Read the model definition and answer for the solid it produces. Units are mm, in the model's axes. Face numbers are marked on the shaded views. A direction names the side the tool comes from. Coordinates: 2 decimals unless noted, no trailing zeros. Write each loop counter-clockwise with the first axis right and the second up, starting at its lowest first coordinate (ties: lowest second). Pieces come first, ordered by that corner, then holes. Notation, with made-up numbers: (42, 24) -> (61, 24) arc R24 cw to (61, 62) -> close; hole circle Ø1 at (44, 72). An arc over 180 degrees is marked (long way). Return JSON: item names as keys, results as strings.
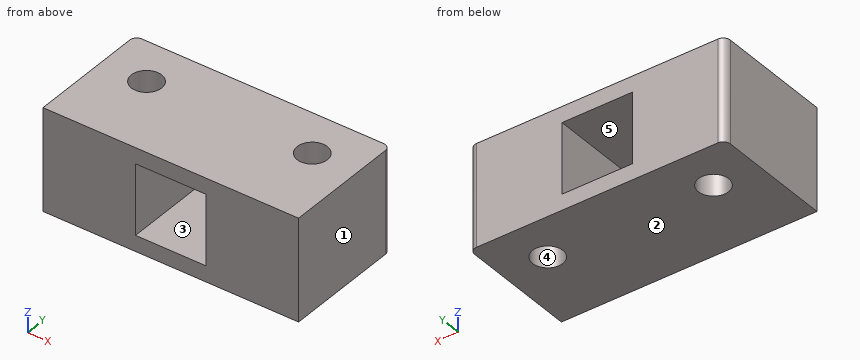
Autodesk Inventor part; units mm, degrees
ref_plane "YZ Plane" through (0, 0, 0) normal (1, 0, 0) x (0, 1, 0)
ref_plane "XZ Plane" through (0, 0, 0) normal (0, 1, 0) x (-1, 0, 0)
ref_plane "XY Plane" through (0, 0, 0) normal (0, 0, 1) x (1, 0, 0)
sketch "Sketch1" plane through (0, 0, 0) normal (0, 0, 1) x (1, 0, 0)
  line L0 (130.1382, 2) -> (130.1382, 24.0208)
  line L1 (114.1591, 40) -> (3.1591, 40)
  line L2 (1.1591, -30) -> (130.1382, -30)
  line L3 (130.1382, -30) -> (130.1382, 2)
  line L4 (1.1591, -30) -> (-14.8135, -30)
  line L5 (-14.8135, -30) -> (-14.8135, 37.6368)
  line L6 (114.1591, 40) -> (126.1382, 40)
  line L7 (130.1382, 36) -> (130.1382, 24.0208)
  line L8 (126.1382, 40) -> (126.1382, 40)
  line L9 (130.1382, 36) -> (130.1382, 36)
  line L10 (-14.8135, 37.6368) -> (-14.8135, 36)
  line L11 (-10.8135, 40) -> (3.1591, 40)
  arc A0 (-10.8135, 40) -> (-14.8135, 36) centre (-10.8135, 36) ccw
  arc A1 (130.1382, 36) -> (126.1382, 40) centre (126.1382, 36) ccw
  circle A2 centre (104.5, 18) radius 8.6
  circle A3 centre (10.5, 18) radius 8.6
  point P0 (130.1382, 40)
  point P1 (-14.8135, 40)
  dimension "d41" = 4
extrude "Extrusion1" add sketch "Sketch1" along normal blind 58 contours L3 L2 L4 L5 A0 L11 L1 L6 A1 L7 L0 | A2 | A3
sketch "Sketch3" plane through (0, 0, 58) normal (0, 0, 1) x (1, 0, 0)
  circle A0 centre (104.5, 18) radius 10.5
  circle A1 centre (10.495, 18) radius 10.5
  point P0 (0, 0)
  dimension "d28" = 21
extrude "Extrusion3" cut sketch "Sketch3" against normal blind 90 contours A1
sketch "Sketch4" plane through (-14.8135, 40, 0) normal (0, 1, 0) x (1, 0, 0)
  line L0 (52.4758, -29) -> (52.4758, -9)
  line L1 (52.4758, -9) -> (72.4758, -9)
  line L2 (52.4758, -9) -> (92.4758, -9)
  line L3 (92.4758, -9) -> (92.4758, -49)
  line L4 (92.4758, -49) -> (52.4758, -49)
  line L5 (52.4758, -49) -> (52.4758, -9)
  point P0 (14.8135, 0)
  dimension "d31" = 20
  dimension "d32" = 20
  dimension "d33" = 40
  dimension "d34" = 40
extrude "Extrusion4" cut sketch "Sketch4" against normal blind 70
sketch "Sketch5" plane through (0, 0, 0) normal (0, 0, -1) x (-1, 0, 0)
  point P0 (0, 0)
sketch "Sketch6" plane through (0, 0, 58) normal (0, 0, 1) x (1, 0, 0)
  circle A0 centre (10.495, 18) radius 10.5
  circle A1 centre (10.495, 18) radius 10.5
  point P0 (0, 0)
extrude "Extrusion5" add sketch "Sketch6" against normal blind 58
sketch "Sketch7" plane through (0, 0, 58) normal (0, 0, 1) x (1, 0, 0)
  line L0 (-14.8135, 36) -> (-14.8135, -30)
  line L1 (130.1382, -30) -> (130.1382, 36)
  line L2 (-14.8135, 14.5974) -> (130.1865, 14.5974)
  line L3 (57.6865, 14.5974) -> (10.684, 14.5974)
  line L4 (10.684, 14.5974) -> (104.689, 14.5974)
  circle A0 centre (104.689, 14.5974) radius 8.6
  circle A1 centre (10.684, 14.5974) radius 8.6
  point P0 (0, 0)
  dimension "d48" = 47.0025
  dimension "d49" = 94.005
  dimension "d50" = 17.2
  dimension "d51" = 17.2
extrude "Extrusion6" cut sketch "Sketch7" against normal blind 58
thread "Thread5"
thread "Thread6"
properties part number "project_rough_mover"
1. Consider L1, parallel to X at y = -7, z = 15; L2, parallel to Z at x = 70.5, y = -24.5; L3, parallel to X at y = 21.5, z = 45.5. Determine where each line is inside the solid, lowest interval first.
Taken from the geometry:
{"L1": "x = -14.81 to 37.66, 77.66 to 130.14", "L2": "z = 0 to 9, 49 to 58", "L3": "x = -14.81 to 5.55, 15.81 to 37.66, 77.66 to 99.56, 109.82 to 130.14"}
2. The part is cut by section C-C (z = 28). Determine the outline of the cut face in (x, y).
Taken from the geometry:
{"outline": "(-14.81, -30) -> (37.66, -30) -> (37.66, 40) -> (-10.81, 40) arc R4 ccw to (-14.81, 36) -> close; (77.66, -30) -> (130.14, -30) -> (130.14, 36) arc R4 ccw to (126.14, 40) -> (77.66, 40) -> close; hole circle Ø17.2 at (10.68, 14.6); hole circle Ø17.2 at (104.69, 14.6)"}
3. For a pull along Z with two mould halves and no side action, classify the marked faces 1, 2 and 3 as +Z half, -Z half, draft (parallel to the pull), parting line (faces both ways), or undercut.
Taken from the geometry:
{"face 1": "draft", "face 2": "-Z half", "face 3": "undercut"}
4. The part is cut by section A-A (x = 68). Determine the outline of the cut face in (y, z).
Taken from the geometry:
{"outline": "(-30, 0) -> (40, 0) -> (40, 9) -> (-30, 9) -> close; (-30, 49) -> (40, 49) -> (40, 58) -> (-30, 58) -> close"}
5. The part is cut by section B-B (y = -15.5). Determine the outline of the cut face in (x, z).
Taken from the geometry:
{"outline": "(-14.81, 0) -> (130.14, 0) -> (130.14, 58) -> (-14.81, 58) -> close; hole (37.66, 9) -> (77.66, 9) -> (77.66, 49) -> (37.66, 49) -> close"}
6. A tool of negligible diameter and unlimited length cuts with its end or side. For the marked faces 4 and 5, from which of +Z, -Z, +X, -X, +Y, -Y can it reach the whole face along a straight path? Write none if from no direction.
Taken from the geometry:
{"face 4": "+Z, -Z", "face 5": "+Y, -Y"}
7. The part is cut by section D-D (y = 21.5). Determine the outline of the cut face in (x, z).
Taken from the geometry:
{"outline": "(-14.81, 0) -> (5.55, 0) -> (5.55, 58) -> (-14.81, 58) -> close; (15.81, 0) -> (99.56, 0) -> (99.56, 58) -> (15.81, 58) -> close; (109.82, 0) -> (130.14, 0) -> (130.14, 58) -> (109.82, 58) -> close; hole (37.66, 9) -> (77.66, 9) -> (77.66, 49) -> (37.66, 49) -> close"}
